from build123d import *

# Parameters (mm, degrees)
BOSS_EXTRUDE1_DEPTH  = 287
M4_CLEARANCE_HOLE1_D = 4.5
M4_CLEARANCE_HOLE2_D = 4.5


with BuildPart() as part:
    # Sketch1 → Boss-Extrude1 (new body)
    with BuildSketch(Plane.XY):
        Polygon((0, 0), (12.7, 0), (12.7, -1.524), (1.524, -1.524), (1.524, -12.7), (0, -12.7), align=None)
    extrude(amount=BOSS_EXTRUDE1_DEPTH)

    # M4 Clearance Hole1 (through all)
    with Locations(Plane(origin=(0, 0, 0), x_dir=(1, 0, 0), z_dir=(0, 1, 0))):
        with Locations((6.35, -7), (6.35, -280), (6.35, -54), (6.35, -76.5)):
            Hole(M4_CLEARANCE_HOLE1_D / 2)

    # M4 Clearance Hole2 (through all)
    with Locations(Plane.ZY):
        with Locations((125, -6.35), (65, -6.35), (185, -6.35)):
            Hole(M4_CLEARANCE_HOLE2_D / 2)


solid = part.part
Build history of the part. All positions in model axes, mm. A direction names the side the tool comes from. Round coordinates to 2 decimals unless told otherwise and drop trailing zeros. Order: outer loops, then holes, each group sorted by start corner. A loop starts at its lowest first (then second) coordinate and runs counter-clockwise, first axis right, second up. Notation, with made-up numbers: M 74.5,12.25 L 133.5,12.25 A27 ccw 133.5,31.25 Z; hole C 82.5,46.5 d3. An arc over 180 degrees is marked long. Use CSV: the item, a comma, the result in double quotes. Start each with the question number.
(1) Flat gauge pins, fed straight in: P1, Ø2.5, axis at x = 6.35, z = 7, coming from the +Y side; P2, Ø1.5, axis at x = 5.5, z = 82.5, coming from the -Y side; P3, Ø6, axis at y = -6.35, z = 125, coming from the +X side. Where does each tip first touch, or does it go through?
(2) Tool access for faces 5 (the face through (0.77, -7.21, 182.92)), 6 (the face through (7, -1.524, 141)): list every direction of +Z, -Z, +X, -X, +Y, -Y with a clear straight run to the whole face (end or side of a thin tool).
(3) Drill centre lines: probe 1 along Z at (x, y) = (6.35, -0.4); probe 2 along X at (y, z) = (-1, 54); probe 3 along Y at (x, z) = (0.7, 65). Where is each one in solid material? Low to high.
(4) Mould opens along Z. For faces 1 (the face through (0.773, -6.251, 67.248)), 2 (the face through (4, -1, 287)), 3 (the face through (1.524, -7, 141)), 4 (the face through (6.838, -0.773, 78.696)) say: +Z half, -Z half, draft (parallel to the pull), parting line (faces both ways), or undercut.
(5) Cut at A-A on z = 198. List the corners of the cut face in (x, y), then the cut area to 3 significant figures.
Findings:
1,P1,"passes through"
1,P2,"stops at y = -1.52"
1,P3,"stops at x = 1.52"
2,face 5,"+X, -X"
2,face 6,"+Z, -Z, +X, -Y"
3,probe 1,"z = 0 to 4.75, 9.25 to 51.75, 56.25 to 74.25, 78.75 to 277.75, 282.25 to 287"
3,probe 2,"x = 0 to 4.1, 8.6 to 12.7"
3,probe 3,"y = -12.7 to -8.6, -4.1 to 0"
4,face 1,"undercut"
4,face 2,"+Z half"
4,face 3,"draft"
4,face 4,"undercut"
5,outline,"M 0,-12.7 L 1.52,-12.7 L 1.52,-1.52 L 12.7,-1.52 L 12.7,0 L 0,0 Z"
5,area,"36.4 mm^2"
